Drawing for the job (mm, zero at the part's lowest x, y, z). A direction names the side the tool comes from. Round coordinates to 2 decimals unless told otherwise and drop trailing zeros. Write each loop counter-clockwise with the first axis right and the second up, starting at its lowest first coordinate (ties: lowest second). Pieces come first, ordered by that corner, then holes. Notation, with made-up numbers: (-29.5, -23) - (12.5, -23) arc R23 cw to (12.5, 7) - close; hole circle Ø9 at (39.5, -14). An arc over 180 degrees is marked (long way). One line per question, with ' | ' between items.
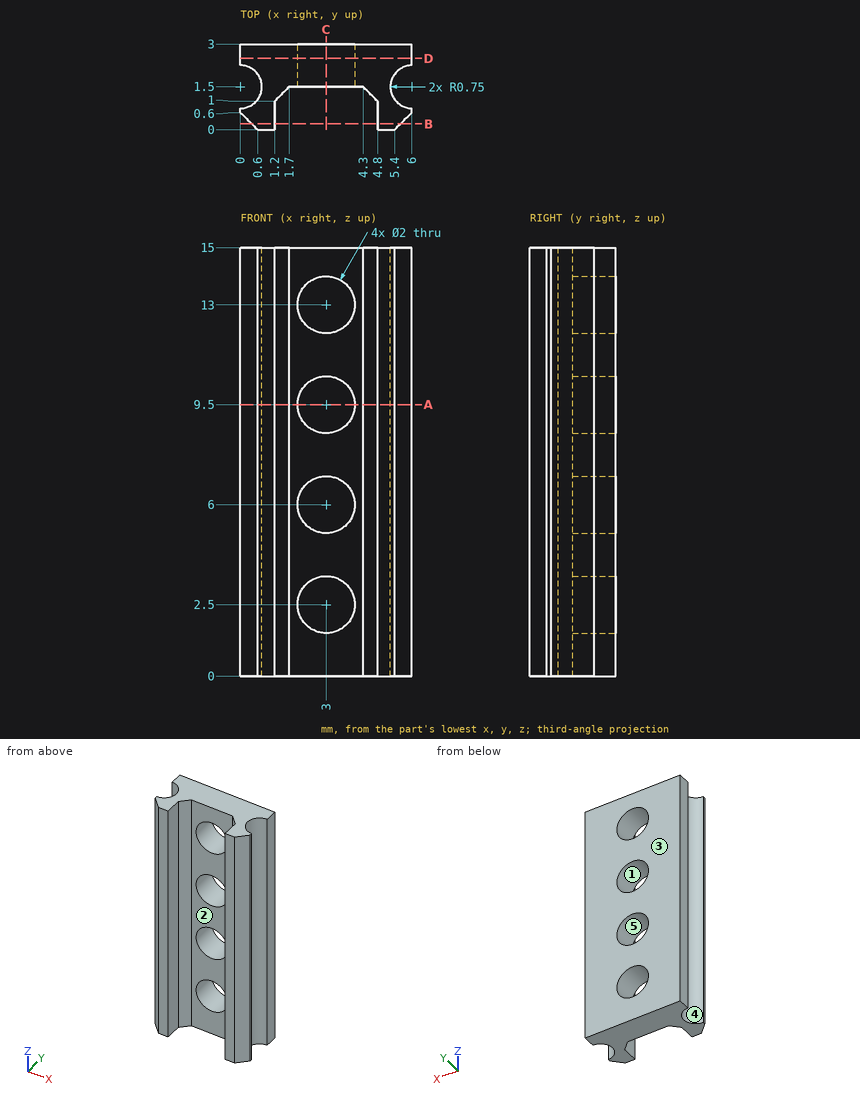
Q1. Drill centre lines: L1, parallel to Z at x = 3, y = 1.8; L2, parallel to X at y = 2.5, z = 6; L3, parallel to X at y = 0.65, z = 9.25. Where is each one in solid material? Low to high. Write a range as from..to.
Found:
L1: 0..1.5, 3.5..5, 7..8.5, 10.5..12, 14..15 | L2: 0..2, 4..6 | L3: 0..1.2, 4.8..6
Q2. Saw through at A-A, the plane z = 9.5. List the corners of the cut face in (x, y).
Found:
outline: (0, 0.6) - (0.6, 0) - (1.2, 0) - (1.2, 1) - (1.7, 1.5) - (2, 1.5) - (2, 3) - (0, 3) - (0, 2.25) arc R0.75 cw to (0, 0.75) - close; (4, 1.5) - (4.3, 1.5) - (4.8, 1) - (4.8, 0) - (5.4, 0) - (6, 0.6) - (6, 0.75) arc R0.75 cw to (6, 2.25) - (6, 3) - (4, 3) - close
Q3. Drop flat-ended pins along their axis: pin 1 (1.6 mm diameter, centred on x = 3, z = 13, fed in from -Y); pin 2 (2 mm diameter, centred on x = 3, z = 5.5, fed in from -Y). Give the stop position or say it passes through.
Found:
pin 1: through | pin 2: y = 1.5
Q4. Saw through at C-C, the plane x = 3. List the corners of the cut face in (y, z), then the cut area to 3 significant figures.
Found:
outline: (1.5, 0) - (3, 0) - (3, 1.5) - (1.5, 1.5) - close; (1.5, 3.5) - (3, 3.5) - (3, 5) - (1.5, 5) - close; (1.5, 7) - (3, 7) - (3, 8.5) - (1.5, 8.5) - close; (1.5, 10.5) - (3, 10.5) - (3, 12) - (1.5, 12) - close; (1.5, 14) - (3, 14) - (3, 15) - (1.5, 15) - close | area: 10.5 mm^2
Q5. Saw through at D-D, the plane y = 2.5. List the corners of the cut face in (x, z), then the cut area to 3 significant figures.
Found:
outline: (0, 0) - (6, 0) - (6, 15) - (0, 15) - close; hole circle Ø2 at (3, 2.5); hole circle Ø2 at (3, 6); hole circle Ø2 at (3, 9.5); hole circle Ø2 at (3, 13) | area: 77.4 mm^2
Q6. Pull direction X, two halves, no side cores. Call the marked faces 3, 4 and 5: +X half, -X half, draft (parallel to the pull), parting line (faces both ways), or undercut.
Found:
face 3: draft | face 4: -X half | face 5: undercut
Q7. Which spindle directions (+Z, -Z, +X, -X, +Y, -Y) get a long thin tool onto all of the face, cutting with end or side? Do the marked faces 1 and 2. Say none if no direction does.
Found:
face 1: +Y, -Y | face 2: +Z, -Z, -Y
Q8. Saw through at B-B, the plane y = 0.2. List the corners of the cut face in (x, z).
Found:
outline: (0.4, 0) - (1.2, 0) - (1.2, 15) - (0.4, 15) - close; (4.8, 0) - (5.6, 0) - (5.6, 15) - (4.8, 15) - close
